Can you work these out from the model? Positions are in its coordinate system, mm. Face numbers are marked on the shaded views. A direction names the side the tool comes from. Coordinates: 2 decimals unless noted, no trailing zeros. Order: outer loops, then holes, each group sorted by start corner. A loop starts at its lowest first (then second) coordinate and runs counter-clockwise, first axis right, second up. Notation, with made-up numbers: (88.5, 59) -> (146.5, 59) arc R21 cw to (146.5, 82) -> close; hole circle Ø11 at (26.25, 56). An arc over 180 degrees is marked (long way). Answer as a JSON object with one key per item and string values. Group by question number.
(1) I want a section at C-C, the plane x = 0. List the corners of the cut face in (y, z) for me, plus the area to 3 significant figures.
(2) I want a section at D-D, the plane y = 5. List the corners of the cut face in (x, z) for me.
(3) If we mould it in two halves opening along X, with no side actions, what happens to the marked faces 1, 2 and 3? For each: pulls with the +X half, pulls with the -X half, needs draft (parallel to the pull), parting line crosses it, or undercut.
(4) I want a section at B-B, the plane y = 2.75. List the corners of the cut face in (x, z) for me, plus the area to 3 significant figures.
(5) I need wall thicknesses on line 1 (X direction, y = 1.75, z = 6); line 2 (Z direction, x = -0.75, y = 1.75); line 3 (X direction, y = 3.25, z = -1.5). Which ranges of each line are inside material? Lowest first, please.
(6) Which directions (+Z, -Z, +X, -X, +Y, -Y) give clear straight access to the entire face, cutting with the end or side of a thin tool? Please do the marked faces 4 and 5.
(7) For pin 1 (1.6 mm diameter, centred on x = 0, z = 6, fed in from +Y); pin 2 (4 mm diameter, centred on x = -1.5, z = -5.5, fed in from +Y), each with a flat end and sliding along its axis, tell me the tip position at first contact or that it passes through.
(8) I want a section at A-A, the plane z = 1. List the corners of the cut face in (x, y) for me.
from build123d import *

# Parameters (mm, degrees)
SKETCH_1_R          = 1.35
EXTRUDE_1_DEPTH     = 3
SKETCH_2_W          = 3
SKETCH_2_H          = 22
EXTRUDE_2_DEPTH     = 7
SKETCH_3_R          = 2
CUT_EXTRUDE_2_DEPTH = 20.104973175
EXTRUDE_3_DEPTH     = 2.5
FILLET_1_R          = 3
CUT_EXTRUDE_3_DEPTH = 1


with BuildPart() as part:
    # Sketch 1 → Extrude 1 (new body)
    with BuildSketch(Plane(origin=(0, 0, 0), x_dir=(1, 0, 0), z_dir=(0, 1, 0))):
        Polygon((-4, -11), (4, -11), (8, -11), (8, 11), (4, 11), (-4, 11), align=None)
        with Locations(Location((0, 6, 0), (0, 0, 270))):
            Circle(SKETCH_1_R, mode=Mode.SUBTRACT)
        with Locations(Location((0, -6, 0), (0, 0, 90))):
            Circle(SKETCH_1_R, mode=Mode.SUBTRACT)
    extrude(amount=EXTRUDE_1_DEPTH)

    # Sketch 2 → Extrude 2 (add)
    with BuildSketch(Plane(origin=(0, 3, 0), x_dir=(1, 0, 0), z_dir=(0, 1, 0))):
        with Locations((6.5, 0)):
            Rectangle(SKETCH_2_W, SKETCH_2_H)
    extrude(amount=EXTRUDE_2_DEPTH)

    # Sketch 3 → Cut-Extrude 2 (cut, through all)
    with BuildSketch(Plane(origin=(8, 0, 0), x_dir=(0, 0, -1), z_dir=(1, 0, 0))):
        with Locations((-1, 6.25)):
            Circle(SKETCH_3_R)
    extrude(amount=-CUT_EXTRUDE_2_DEPTH, mode=Mode.SUBTRACT)

    # Sketch 4 → Extrude 3 (add)
    with BuildSketch(Plane(origin=(0, 0, -11), x_dir=(-1, 0, 0), z_dir=(0, 0, -1))):
        Polygon((-5, 10), (-5, 3), (4, 3), align=None)
    extrude_3 = extrude(amount=-EXTRUDE_3_DEPTH)

    # Mirror 1: Extrude 3 across plane
    add(extrude_3.mirror(Plane.XY))

    # Fillet 1
    fillet_1_edges = [part.edges().sort_by_distance(p)[0] for p in [
        (5, 6.5, -8.5),
        (5, 6.5, 8.5),
    ]]
    fillet(fillet_1_edges, radius=FILLET_1_R)

    # Sketch 5 → Cut-Extrude 3 (cut)
    with BuildSketch(Plane(origin=(0, 3, 0), x_dir=(1, 0, 0), z_dir=(0, 1, 0))):
        Polygon((1.5, 2.25), (5, 2.25), (5, -4.25), (1.5, -4.25), (1.5, -3), (-4, -3), (-4, 1), (1.5, 1), align=None)
    extrude(amount=-CUT_EXTRUDE_3_DEPTH, mode=Mode.SUBTRACT)


solid = part.part
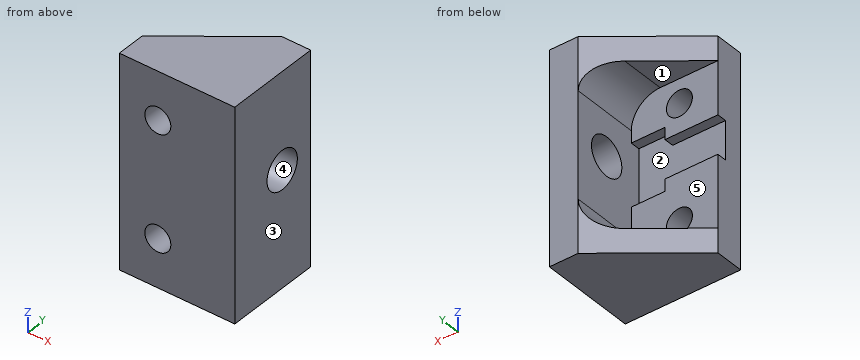
Computed values:
{
 "1": {"outline": "(0, -11) -> (6.11, -11) -> (6.11, -8.5) -> (3, -8.5) -> (3, -7.35) -> (0, -7.35) -> close; (0, -4.65) -> (3, -4.65) -> (3, -1) -> (2, -1) -> (2, 3) -> (3, 3) -> (3, 4.65) -> (0, 4.65) -> close; (0, 7.35) -> (3, 7.35) -> (3, 8.5) -> (6.11, 8.5) -> (6.11, 11) -> (0, 11) -> close", "area": "61.4 mm2"},
 "2": {"outline": "(-1.43, -11) -> (8, -11) -> (8, -0.56) -> (5, -0.56) -> (5, -5.5) arc R3 cw to (2, -8.5) -> (-1.43, -8.5) -> close; (-1.43, 8.5) -> (2, 8.5) arc R3 cw to (5, 5.5) -> (5, 2.56) -> (8, 2.56) -> (8, 11) -> (-1.43, 11) -> close"},
 "3": {"face 1": "needs draft", "face 2": "undercut", "face 3": "pulls with the +X half"},
 "4": {"outline": "(-4, -11) -> (8, -11) -> (8, 11) -> (-4, 11) -> (-4, 3) -> (1.5, 3) -> (1.5, 4.25) -> (5, 4.25) -> (5, -2.25) -> (1.5, -2.25) -> (1.5, -1) -> (-4, -1) -> close; hole circle Ø2.7 at (0, -6); hole circle Ø2.7 at (0, 6)", "area": "208 mm2"},
 "5": {"line 1": "x = -4 to -1.35, 1.35 to 8", "line 2": "z = -11 to -7.12, -4.88 to 4.88, 7.12 to 11", "line 3": "x = 5 to 8"},
 "6": {"face 4": "+X, -X", "face 5": "-X, +Y"},
 "7": {"pin 1": "passes through", "pin 2": "stops at y = 3"},
 "8": {"outline": "(-4, 0) -> (8, 0) -> (8, 4.25) -> (5, 4.25) -> (5, 2) -> (-4, 2) -> close; (5, 8.25) -> (8, 8.25) -> (8, 10) -> (5, 10) -> close"}
}
